from build123d import *

# Parameters (mm, degrees)
SKETCH1_R           = 2.1
BOSS_EXTRUDE1_DEPTH = 960


with BuildPart() as part:
    # Sketch1 → Boss-Extrude1 (new body)
    with BuildSketch(Plane.XY.offset(1000)):
        with BuildLine():
            Line((6.560660172, 4.5), (3.9, 7.160660172))
            Line((3.9, 7.160660172), (3.9, 9.79))
            Line((3.9, 9.79), (3.69, 10))
            Line((3.69, 10), (3.9, 10.21))
            Line((3.9, 10.21), (3.9, 12.839339828))
            Line((3.9, 12.839339828), (6.560660172, 15.5))
            Line((6.560660172, 15.5), (8.2, 15.5))
            Line((8.2, 15.5), (8.2, 13.125))
            Line((8.2, 13.125), (8.545, 13.125))
            Line((8.545, 13.125), (10, 14.58))
            Line((10, 14.58), (10, 19.5))
            ThreePointArc((10, 19.5), (9.853553391, 19.853553391), (9.5, 20))
            Line((9.5, 20), (4.58, 20))
            Line((4.58, 20), (3.125, 18.545))
            Line((3.125, 18.545), (3.125, 18.2))
            Line((3.125, 18.2), (5.5, 18.2))
            Line((5.5, 18.2), (5.5, 16.560660172))
            Line((5.5, 16.560660172), (2.839339828, 13.9))
            Line((2.839339828, 13.9), (0.21, 13.9))
            Line((0.21, 13.9), (0, 13.69))
            Line((0, 13.69), (-0.21, 13.9))
            Line((-0.21, 13.9), (-2.839339828, 13.9))
            Line((-2.839339828, 13.9), (-5.5, 16.560660172))
            Line((-5.5, 16.560660172), (-5.5, 18.2))
            Line((-5.5, 18.2), (-3.125, 18.2))
            Line((-3.125, 18.2), (-3.125, 18.545))
            Line((-3.125, 18.545), (-4.58, 20))
            Line((-4.58, 20), (-9.5, 20))
            ThreePointArc((-9.5, 20), (-9.853553391, 19.853553391), (-10, 19.5))
            Line((-10, 19.5), (-10, 14.58))
            Line((-10, 14.58), (-8.545, 13.125))
            Line((-8.545, 13.125), (-8.2, 13.125))
            Line((-8.2, 13.125), (-8.2, 15.5))
            Line((-8.2, 15.5), (-6.560660172, 15.5))
            Line((-6.560660172, 15.5), (-3.9, 12.839339828))
            Line((-3.9, 12.839339828), (-3.9, 10.21))
            Line((-3.9, 10.21), (-3.69, 10))
            Line((-3.69, 10), (-3.9, 9.79))
            Line((-3.9, 9.79), (-3.9, 7.160660172))
            Line((-3.9, 7.160660172), (-6.560660172, 4.5))
            Line((-6.560660172, 4.5), (-8.2, 4.5))
            Line((-8.2, 4.5), (-8.2, 6.875))
            Line((-8.2, 6.875), (-8.545, 6.875))
            Line((-8.545, 6.875), (-10, 5.42))
            Line((-10, 5.42), (-10, -5.42))
            Line((-10, -5.42), (-8.545, -6.875))
            Line((-8.545, -6.875), (-8.2, -6.875))
            Line((-8.2, -6.875), (-8.2, -4.5))
            Line((-8.2, -4.5), (-6.560660172, -4.5))
            Line((-6.560660172, -4.5), (-3.9, -7.160660172))
            Line((-3.9, -7.160660172), (-3.9, -9.79))
            Line((-3.9, -9.79), (-3.69, -10))
            Line((-3.69, -10), (-3.9, -10.21))
            Line((-3.9, -10.21), (-3.9, -12.839339828))
            Line((-3.9, -12.839339828), (-6.560660172, -15.5))
            Line((-6.560660172, -15.5), (-8.2, -15.5))
            Line((-8.2, -15.5), (-8.2, -13.125))
            Line((-8.2, -13.125), (-8.545, -13.125))
            Line((-8.545, -13.125), (-10, -14.58))
            Line((-10, -14.58), (-10, -19.5))
            ThreePointArc((-10, -19.5), (-9.853553391, -19.853553391), (-9.5, -20))
            Line((-9.5, -20), (-4.58, -20))
            Line((-4.58, -20), (-3.125, -18.545))
            Line((-3.125, -18.545), (-3.125, -18.2))
            Line((-3.125, -18.2), (-5.5, -18.2))
            Line((-5.5, -18.2), (-5.5, -16.560660172))
            Line((-5.5, -16.560660172), (-2.839339828, -13.9))
            Line((-2.839339828, -13.9), (-0.21, -13.9))
            Line((-0.21, -13.9), (0, -13.69))
            Line((0, -13.69), (0.21, -13.9))
            Line((0.21, -13.9), (2.839339828, -13.9))
            Line((2.839339828, -13.9), (5.5, -16.560660172))
            Line((5.5, -16.560660172), (5.5, -18.2))
            Line((5.5, -18.2), (3.125, -18.2))
            Line((3.125, -18.2), (3.125, -18.545))
            Line((3.125, -18.545), (4.58, -20))
            Line((4.58, -20), (9.5, -20))
            ThreePointArc((9.5, -20), (9.853553391, -19.853553391), (10, -19.5))
            Line((10, -19.5), (10, -14.58))
            Line((10, -14.58), (8.545, -13.125))
            Line((8.545, -13.125), (8.2, -13.125))
            Line((8.2, -13.125), (8.2, -15.5))
            Line((8.2, -15.5), (6.560660172, -15.5))
            Line((6.560660172, -15.5), (3.9, -12.839339828))
            Line((3.9, -12.839339828), (3.9, -10.21))
            Line((3.9, -10.21), (3.69, -10))
            Line((3.69, -10), (3.9, -9.79))
            Line((3.9, -9.79), (3.9, -7.160660172))
            Line((3.9, -7.160660172), (6.560660172, -4.5))
            Line((6.560660172, -4.5), (8.2, -4.5))
            Line((8.2, -4.5), (8.2, -6.875))
            Line((8.2, -6.875), (8.545, -6.875))
            Line((8.545, -6.875), (10, -5.42))
            Line((10, -5.42), (10, 5.42))
            Line((10, 5.42), (8.545, 6.875))
            Line((8.545, 6.875), (8.2, 6.875))
            Line((8.2, 6.875), (8.2, 4.5))
            Line((8.2, 4.5), (6.560660172, 4.5))
        make_face()
        with Locations(Location((0, 10, 0), (0, 0, 180))):
            Circle(SKETCH1_R, mode=Mode.SUBTRACT)
        with Locations(Location((0, -10, 0), (0, 0, 180))):
            Circle(SKETCH1_R, mode=Mode.SUBTRACT)
        Polygon((2.839339828, -6.1), (-2.839339828, -6.1), (-6.239339828, -2.7), (-8.2, -2.7), (-8.2, 2.7), (-6.239339828, 2.7), (-2.839339828, 6.1), (2.839339828, 6.1), (6.239339828, 2.7), (8.2, 2.7), (8.2, -2.7), (6.239339828, -2.7), align=None, mode=Mode.SUBTRACT)
    extrude(amount=-BOSS_EXTRUDE1_DEPTH)


solid = part.part
Work out the finished part from the listing and answer in its coordinate system (mm). Coordinates: 2 decimals unless noted, no trailing zeros. Write item = value, one per line.
1. Flat-ended cylindrical pins translate along their axes: pin 1 (8 mm diameter, centred on x = -5, y = 1, fed in from -Z); pin 2 (0.8 mm diameter, centred on y = 8.5, z = 503, fed in from -X); pin 3 (1 mm diameter, centred on x = 0.5, z = 770, fed in from +Y); pin 4 (4 mm diameter, centred on x = 7.5, y = 10.5, fed in from -Z). Find the tip coordinate at first contact, or state that the pin passes through.
Solution:
pin_1 = 40
pin_2 = -3.9
pin_3 = 13.9
pin_4 = through
2. Straight lines are drawn through the part: line 1 (Y direction, x = 0, z = 373.5); line 2 (Y direction, x = 8, z = 785); line 3 (Y direction, x = 8.5, z = 373.5) (3 decimals). For each, find the intervals that lie inside material, in ascending order. Write a range as from..to.
Solution:
line_1 = -13.69..-12.1, -7.9..-6.1, 6.1..7.9, 12.1..13.69
line_2 = -20..-15.5, -4.5..-2.7, 2.7..4.5, 15.5..20
line_3 = -20..-13.125, -6.875..6.875, 13.125..20
3. The part is cut by section A-A (z = 541). State how many separate pieces and enclosed holes the cut face has, then the cut area to 3 significant figures.
Solution:
separate_pieces = 1
enclosed_holes = 3
area = 300 mm2
